Input: part model. Units: mm. Frame: model coordinates. A direction names the side the tool comes from. Coordinates: 2 decimals unless noted, no trailing zeros. Write each loop counter-clockwise with the first axis right and the second up, starting at its lowest first coordinate (ties: lowest second). Pieces come first, ordered by that corner, then holes. Notation, with made-up numbers: (-35.75, 86) - (8.25, 86) arc R15 ccw to (8.25, 109) - close; hole circle Ø4 at (-36, 86.5). An arc over 180 degrees is marked (long way). Use a Markdown table: item, result. Add a question column.
Q1. Material intervals for probe 1 along X at (y, z) = (-0.95, 0.9); probe 2 along Z at (x, y) = (9, 0.15); probe 3 along X at (y, z) = (-1.45, -0.95), sorted ascending. Write a range as from..to.
Q2. Pin query (flat end, axial travel): P1, Ø2, axis at x = 20, z = 1, coming from the +Y side; P2, Ø2, axis at x = 10.5, y = -1, coming from the -Z side. Return the tip coordinate at first contact, or that it passes through.
Q3. Set-up query: faces 1 (the face through (-1, 2, 0)), 2 (the face through (-6.75, -0.5, -0.5)). Return all of +Z, -Z, +X, -X, +Y, -Y with unobstructed straight access to the full face (end or side cutting, diameter ignored); none if empty.
Q4. Section query A-A (x = -25). Return the cut outline in (y, z).
from build123d import *


with BuildPart() as f1:
    # F0 (on Front) → F1 (revolve)
    with BuildSketch(Plane.XZ):
        with BuildLine():
            Line((-40.6, 0.5), (-40.6, 0))
            Line((-40.6, 0), (-6.75, 0))
            Line((-6.75, 0), (0, 0))
            Line((0, 0), (6.75, 0))
            Line((6.75, 0), (40.6, 0))
            Line((40.6, 0), (40.6, 0.5))
            Line((40.6, 0.5), (6.75, 0.5))
            ThreePointArc((6.75, 0.5), (5.566246, 1.600617), (4, 2))
            Line((4, 2), (0, 2))
            Line((0, 2), (-6.75, 2))
            Line((-6.75, 2), (-6.75, 0.5))
            Line((-6.75, 0.5), (-40.6, 0.5))
        make_face()
    revolve(axis=Axis((-3.375, 0, 0), (1, 0, 0)))


solid = f1.part
Values follow:
| question | item | result |
|---|---|---|
| 1 | probe 1 | -6.75..6.01 |
| 1 | probe 2 | -0.48..0.48 |
| 1 | probe 3 | -6.75..5.29 |
| 2 | P1 | y = 0.5 |
| 2 | P2 | z = -0.5 |
| 3 | face 1 | +X, -X |
| 3 | face 2 | -X |
| 4 | outline | circle Ø1 at (0, 0) |
